Here's how the part is built. I have some questions about the finished solid (model axes, mm). A direction names the side the tool comes from. Give positions to 0.01 mm unless a question says otherwise; leave off trailing zeros. Loops run counter-clockwise (first coordinate to the right, second up) from the corner with the lowest first, then second, coordinate; pieces in that order, holes last. Notation, with made-up numbers: (44.5, 4) - (56.5, 4) arc R29 ccw to (56.5, 24) - close; hole circle Ø5 at (31.5, -24). An arc over 180 degrees is marked (long way). Return JSON: item names as keys, results as strings. Group by question number.
(1) I need wall thicknesses on probe 1 along Y at (x, z) = (5.5, 24.5); probe 2 along Y at (x, z) = (18, 7); probe 3 along X at (y, z) = (-54.5, 6.5). Which ranges of each line are inside material? Lowest first, please. Write a range as [from, to].
(2) If we section it at C-C (y = -69): Please give me the cut outline in (x, z).
(3) If we section it at B-B (z = 0): Please give me the cut outline in (x, y).
(4) If we section it at A-A (x = 0): Please give me the cut outline in (y, z), then the cut area to 3 significant figures.
(5) On a 3-axis mill with a long thin cutter (end or side, diameter ignored), from which of +Z, -Z, +X, -X, +Y, -Y can I reach the whole of each face in a straight line? I mean faces 1 (the cylindrical face through (19.524, 15.605, 4.336)), 2 (the cylindrical face through (-3.47, -49.05, 15.62)), 3 (the cylindrical face through (21, 4, 28)). Say none if no direction works.
(6) For P1, Ø6, axis at x = 25.5, z = 8, coming from the +Y side; P2, Ø12, axis at x = 0.5, y = -62.5, coming from the -Z side; P3, Ø3, axis at y = -20, z = -9.5, coming from the -X side, each with a flat end and sliding along its axis, tell me the tip position at first contact or that it passes through.
Autodesk Inventor part; units mm, degrees
ref_plane "YZ Plane" through (0, 0, 0) normal (1, 0, 0) x (0, 1, 0)
ref_plane "XZ Plane" through (0, 0, 0) normal (0, 1, 0) x (-1, 0, 0)
ref_plane "XY Plane" through (0, 0, 0) normal (0, 0, 1) x (1, 0, 0)
sketch "Skizze1" plane through (0, 0, 0) normal (1, 0, 0) x (0, 1, 0)
  line L0 (8, 0) -> (0, 0)
  line L1 (0, 0) -> (0, -35)
  line L2 (0, -35) -> (8, -35)
  line L3 (8, -35) -> (8, 0)
  line L4 (23, 0) -> (8, 0)
  line L5 (8, 0) -> (8, -20)
  line L6 (8, -20) -> (23, -20)
  line L7 (23, -20) -> (23, 0)
  dimension "d0" = 20
  dimension "d1" = 35
  dimension "d2" = 8
  dimension "d3" = 15
revolve "Umdrehung1" add sketch "Skizze1" angle 360 about axis through (0, 23, 0) along (0, -1, 0)
chamfer "Fase1" distance 0.25 angle 45 2 edges at (0, 8, 35) (0, 0, 35)
sketch "Skizze2" plane through (0, 0, 0) normal (0, -1, 0) x (1, 0, 0)
  circle A0 centre (0, 0) radius 16
  dimension "d8" = 32
extrude "Extrusion1" add sketch "Skizze2" along normal blind 100
chamfer "Fase2" distance 0.5 angle 45 1 edges at (-16, -100, 0)
properties part number "Stempel"
Values:
{
 "1": {"probe 1": "[0, 8]", "probe 2": "[0, 23]", "probe 3": "[-14.62, 14.62]"},
 "2": {"outline": "circle Ø32 at (0, 0)"},
 "3": {"outline": "(-35, 0.25) - (-34.75, 0) - (-16, 0) - (-16, -99.5) - (-15.5, -100) - (15.5, -100) - (16, -99.5) - (16, 0) - (34.75, 0) - (35, 0.25) - (35, 7.75) - (34.75, 8) - (20, 8) - (20, 23) - (-20, 23) - (-20, 8) - (-34.75, 8) - (-35, 7.75) - close"},
 "4": {"outline": "(-100, -15.5) - (-99.5, -16) - (0, -16) - (0, -34.75) - (0.25, -35) - (7.75, -35) - (8, -34.75) - (8, -20) - (23, -20) - (23, 20) - (8, 20) - (8, 34.75) - (7.75, 35) - (0.25, 35) - (0, 34.75) - (0, 16) - (-99.5, 16) - (-100, 15.5) - close", "area": "4,360 mm2"},
 "5": {"face 1": "+Y", "face 2": "-Y", "face 3": "+Y, -Y"},
 "6": {"P1": "y = 8", "P2": "z = -16", "P3": "x = -13.86"}
}
